```python
from build123d import *

# Parameters (mm, degrees)
F0_W     = 101.6
F0_H     = 177.8
F1_DEPTH = 50.8
F2_T     = -6.35
F3_W     = 152.4
F3_H     = 76.2
F4_DEPTH = 25.4
F5_W     = 152.4
F5_H     = 76.2
F6_DEPTH = 25.4
F7_R     = 12.7
F8_DEPTH = 88.9


with BuildPart() as f1:
    # F0 (on Top) → F1 (new body, symmetric)
    with BuildSketch(Plane.XY):
        Rectangle(F0_W, F0_H)
    extrude(amount=F1_DEPTH, both=True)

    # F2
    f2_openings = [f1.faces().sort_by_distance(p)[0] for p in [
        (0, 0, 50.8),
    ]]
    offset(amount=F2_T, openings=f2_openings)

    # F3 (on face) → F4 (join)
    with BuildSketch(Plane.YZ.offset(50.8)):
        Rectangle(F3_W, F3_H)
    extrude(amount=F4_DEPTH)

    # F5 (on face) → F6 (join)
    with BuildSketch(Plane(origin=(-50.8, 0, 0), x_dir=(0, -1, 0), z_dir=(-1, 0, 0))):
        Rectangle(F5_W, F5_H)
    extrude(amount=F6_DEPTH)

    # F7 (on face) → F8 (join)
    with BuildSketch(Plane(origin=(44.45, 0, 0), x_dir=(0, -1, 0), z_dir=(-1, 0, 0))):
        with Locations((-63.5, -25.4)):
            Circle(F7_R)
    extrude(amount=F8_DEPTH)


solid = f1.part
```
Geometry: final body of the model. Coordinates: model frame, mm. A direction names the side the tool comes from. Round coordinates to 2 decimals unless told otherwise and drop trailing zeros. Loops run counter-clockwise (first coordinate to the right, second up) from the corner with the lowest first, then second, coordinate; pieces in that order, holes last. Notation, with made-up numbers: (7.25, 34.5) -> (45.25, 34.5) arc R21 ccw to (45.25, 61.5) -> close; hole circle Ø3 at (66, 55). An arc over 180 degrees is marked (long way). Write each question's results on one line, items separated by ' | '.
Item 1: Pull-direction query (Y, two-part tool) for faces 6 (the face through (-50.8, -1, -44)), 7 (the face through (63, 76.2, -1)), 8 (the face through (-1, 82.55, 4)); classes: pulls with the +Y half, pulls with the -Y half, needs draft (parallel to the pull), parting line crosses it, or undercut.
Answers below:
face 6: needs draft | face 7: pulls with the +Y half | face 8: undercut
Item 2: Line query: probe 1 along Y at (x, z) = (2, -26); probe 2 along Y at (x, z) = (32.5, 33); probe 3 along X at (y, z) = (-71.5, -16). Output: solid intervals per line, ascending. Write a range as [from, to].
Answers below:
probe 1: y = [-88.9, -82.55], [50.81, 76.19], [82.55, 88.9] | probe 2: y = [-88.9, -82.55], [82.55, 88.9] | probe 3: x = [-76.2, -44.45], [44.45, 76.2]
Item 3: Cut plane C-C on y = 63.5. Return the cut outline in (x, z).
Answers below:
outline: (-76.2, -38.1) -> (-50.8, -38.1) -> (-50.8, -50.8) -> (50.8, -50.8) -> (50.8, -38.1) -> (76.2, -38.1) -> (76.2, 38.1) -> (50.8, 38.1) -> (50.8, 50.8) -> (44.45, 50.8) -> (44.45, -12.7) -> (-44.45, -12.7) -> (-44.45, 50.8) -> (-50.8, 50.8) -> (-50.8, 38.1) -> (-76.2, 38.1) -> close; hole (-44.45, -44.45) -> (44.45, -44.45) -> (44.45, -38.1) -> (-44.45, -38.1) -> close
Item 4: Pin query (flat end, axial travel): pin 1 Ø7.5 at (x, y) = (59.5, -33) entering from -Z; pin 2 Ø12.5 at (x, z) = (64.5, -6.5) entering from -Y; pin 3 Ø20.5 at (x, z) = (-60.5, -11.5) entering from +Y; pin 4 Ø2 at (x, y) = (8.5, -38) entering from +Z. Return the tip coordinate at first contact, or that it passes through.
Answers below:
pin 1: stops at z = -38.1 | pin 2: stops at y = -76.2 | pin 3: stops at y = 88.9 | pin 4: stops at z = -44.45
Item 5: Cut plane A-A on x = -34. Return the cut outline in (y, z), and give its area (3 significant figures).
Answers below:
outline: (-88.9, -50.8) -> (88.9, -50.8) -> (88.9, 50.8) -> (82.55, 50.8) -> (82.55, -44.45) -> (-82.55, -44.45) -> (-82.55, 50.8) -> (-88.9, 50.8) -> close; circle Ø25.4 at (63.5, -25.4) | area: 2,850 mm²
Item 6: Cut plane D-D on z = -41. Return the cut outline in (x, y).
Answers below:
outline: (-50.8, -88.9) -> (50.8, -88.9) -> (50.8, 88.9) -> (-50.8, 88.9) -> close; hole (-44.45, -82.55) -> (44.45, -82.55) -> (44.45, 82.55) -> (-44.45, 82.55) -> close
Item 7: Cut plane B-B on z = -25.4. Return the cut outline in (x, y), and give its area (3 significant figures).
Answers below:
outline: (-76.2, -76.2) -> (-50.8, -76.2) -> (-50.8, -88.9) -> (50.8, -88.9) -> (50.8, -76.2) -> (76.2, -76.2) -> (76.2, 76.2) -> (50.8, 76.2) -> (50.8, 88.9) -> (-50.8, 88.9) -> (-50.8, 76.2) -> (-76.2, 76.2) -> close; hole (-44.45, -82.55) -> (44.45, -82.55) -> (44.45, 50.8) -> (-44.45, 50.8) -> close; hole (-44.45, 76.2) -> (44.45, 76.2) -> (44.45, 82.55) -> (-44.45, 82.55) -> close | area: 13,400 mm²
Item 8: Set-up query: faces 1 (the face through (63, -76.2, -1)), 2 (the face through (63, -1, 38.1)), 3 (the face through (-63, 1, -38.1)), 4 (the face through (-63, 76.2, -1)), 5 (the face through (-63, -76.2, -1)). Return all of +Z, -Z, +X, -X, +Y, -Y with unobstructed straight access to the full face (end or side cutting, diameter ignored); none if empty.
Answers below:
face 1: +Z, -Z, +X, -Y | face 2: +Z, +X, +Y, -Y | face 3: -Z, -X, +Y, -Y | face 4: +Z, -Z, -X, +Y | face 5: +Z, -Z, -X, -Y
